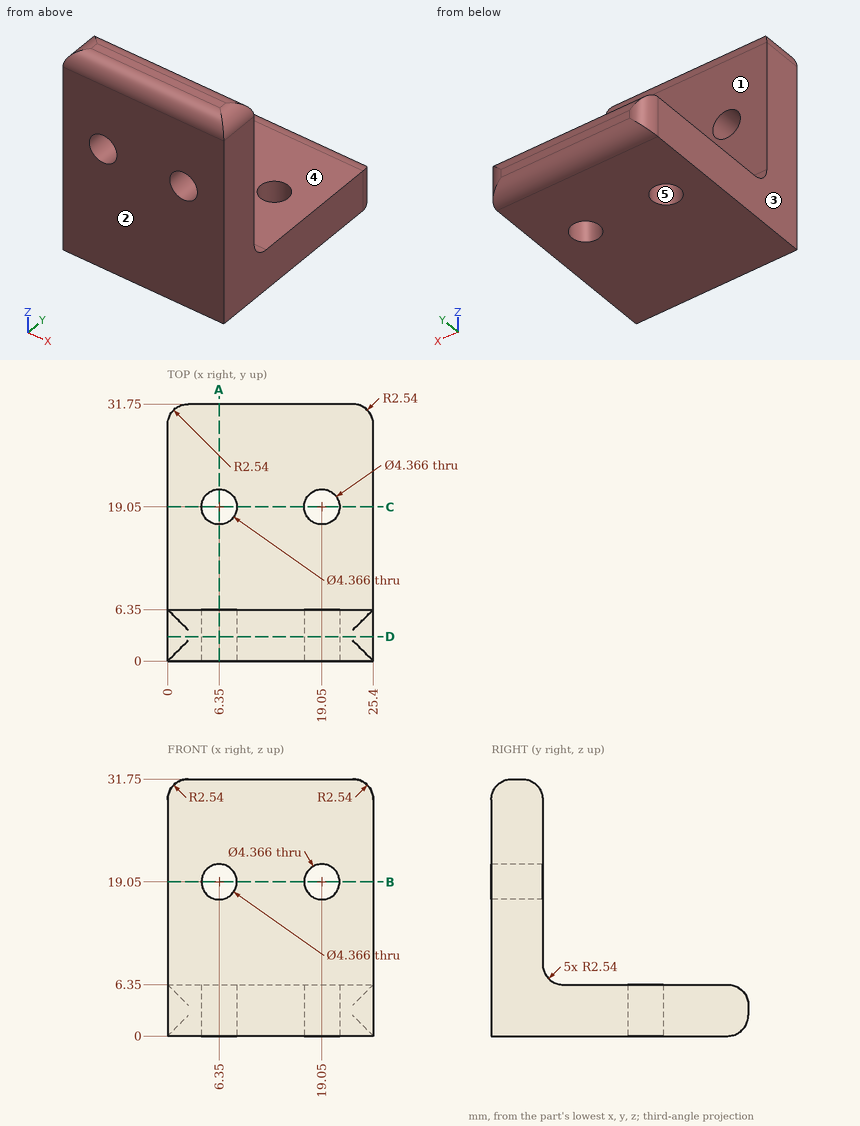
Input: dimensioned drawing with shaded views. Units: mm. Origin: part minimum x, y, z. A direction names the side the tool comes from. Round coordinates to 2 decimals unless told otherwise and drop trailing zeros. Order: outer loops, then holes, each group sorted by start corner. A loop starts at its lowest first (then second) coordinate and runs counter-clockwise, first axis right, second up. Notation, with made-up numbers: (-2, 61) -> (57, 61) arc R25 cw to (57, 95) -> close; hole circle Ø6 at (43, 10.25). An arc over 180 degrees is marked (long way). One line per item, written item: value. Start each with the question number.
Q1. Draft query along X for the marked faces 3, 4 and 5. Return one class per face: pulls with the +X half, pulls with the -X half, needs draft (parallel to the pull), parting line crosses it, or undercut.
Q2. Section query D-D (y = 3). Return the cut outline in (x, z), plus the area to 3 significant figures.
Q3. Access query for the marked faces 1 and 2. Directions: +Z, -Z, +X, -X, +Y, -Y. A direction counts if a zero-diameter tool reaches every point of the face in a straight line with its end or side. Return the directions, or none.
Q4. Material intervals for probe 1 along X at (y, z) = (3.5, 19.05); probe 2 along Y at (x, z) = (6.35, 3.75); probe 3 along Y at (x, z) = (16.5, 27.5), sorted ascending.
Q5. Section query A-A (x = 6.35). Return the cut outline in (y, z), plus the area to 3 significant figures.
Q6. Section query B-B (z = 19.05). Return the cut outline in (x, y), plus the area to 3 significant figures.
Q7. Pin query (flat end, axial travel): pin 1 (4 mm diameter, centred on x = 19, y = 28, fed in from +Z); pin 2 (10 mm diameter, centred on y = 26.5, z = 12.5, fed in from +X); pin 3 (2 mm diameter, centred on x = 9, z = 20.5, fed in from +Y). Return the tip coordinate at first contact, or that it passes through.
Findings below:
1. face 3: pulls with the -X half
1. face 4: needs draft
1. face 5: undercut
2. outline: (0, 0) -> (25.4, 0) -> (25.4, 29.21) arc R2.54 ccw to (22.86, 31.75) -> (2.54, 31.75) arc R2.54 ccw to (0, 29.21) -> close; hole circle Ø4.37 at (6.35, 19.05); hole circle Ø4.37 at (19.05, 19.05)
2. area: 774 mm²
3. face 1: +Z, +X, -X, +Y
3. face 2: +Z, -Z, +X, -X, -Y
4. probe 1: 0 to 4.17, 8.53 to 16.87, 21.23 to 25.4
4. probe 2: 0 to 16.87, 21.23 to 31.75
4. probe 3: 0 to 6.35
5. outline: (0, 0) -> (16.87, 0) -> (16.87, 6.35) -> (8.89, 6.35) arc R2.54 cw to (6.35, 8.89) -> (6.35, 16.87) -> (0, 16.87) -> close; (0, 21.23) -> (6.35, 21.23) -> (6.35, 29.21) arc R2.54 ccw to (3.81, 31.75) -> (2.54, 31.75) arc R2.54 ccw to (0, 29.21) -> close; (21.23, 0) -> (29.21, 0) arc R2.54 ccw to (31.75, 2.54) -> (31.75, 3.81) arc R2.54 ccw to (29.21, 6.35) -> (21.23, 6.35) -> close
5. area: 303 mm²
6. outline: (0, 0) -> (4.17, 0) -> (4.17, 6.35) -> (0, 6.35) -> close; (8.53, 0) -> (16.87, 0) -> (16.87, 6.35) -> (8.53, 6.35) -> close; (21.23, 0) -> (25.4, 0) -> (25.4, 6.35) -> (21.23, 6.35) -> close
6. area: 106 mm²
7. pin 1: z = 6.35
7. pin 2: through
7. pin 3: y = 6.35
